```python
from build123d import *

# Parameters (mm, degrees)
SKETCH1_R                                      = 40
SKETCH1_R_2                                    = 20
BOSS_EXTRUDE1_DEPTH                            = 8.5
SKETCH2_R                                      = 1
CUT_EXTRUDE2_DEPTH                             = 58.203583804
SKETCH2_6_R                                    = 3
SKETCH2_6_R_2                                  = 1
BOSS_EXTRUDE3_DEPTH                            = 8.5
CIRPATTERN1_COUNT                              = 4
CUT_EXTRUDE4_DEPTH                             = 62.402361518
CIRPATTERN3_COUNT                              = 4
SKETCH7_R                                      = 21
CUT_EXTRUDE5_DEPTH                             = 7
SKETCH8_R                                      = 1
OUTER_RETAINER_M2_TAPPED_ENVELOPE_DEPTH        = 4.3
SKETCH9_R                                      = 1
REVB_OLDHAM_FOUR_M2_BLIND_THREAD_MAJOR_DEPTH   = 5.8
SKETCH10_R                                     = 1.51
REVB_OLDHAM_FOUR_D3P02_PILOT_POCKETS_DEPTH     = 1.1
SKETCH11_R                                     = 1.05
BENCH_OUTERRETAINER_M2_THREAD_MAJOR_ENVE_DEPTH = 4
SKETCH12_R                                     = 1.05
BENCH_OLDHAM_M2_CLEARANCE_4X_D2P1_DEPTH        = 9


with BuildPart() as part:
    # Sketch1 → Boss-Extrude1 (new body)
    with BuildSketch(Plane(origin=(0, 0, 0), x_dir=(1, 0, 0), z_dir=(0, 1, 0))):
        with Locations(Location((0, 0, 0), (0, 0, 270))):
            Circle(SKETCH1_R)
        with Locations(Location((0, 0, 0), (0, 0, 270))):
            Circle(SKETCH1_R_2, mode=Mode.SUBTRACT)
    extrude(amount=BOSS_EXTRUDE1_DEPTH)

    # Sketch2 → Cut-Extrude2 (cut, through all)
    with BuildSketch(Plane(origin=(0, 8.5, 0), x_dir=(1, 0, 0), z_dir=(0, 1, 0))):
        with Locations((40, 0)):
            Circle(SKETCH2_R)
    cut_extrude2 = extrude(amount=-CUT_EXTRUDE2_DEPTH, mode=Mode.SUBTRACT)

    # Sketch2_6 → Boss-Extrude3 (add)
    with BuildSketch(Plane(origin=(0, 8.5, 0), x_dir=(1, 0, 0), z_dir=(0, 1, 0))):
        with Locations((40, 0)):
            Circle(SKETCH2_6_R)
        with Locations(Location((40, 0, 0), (0, 0, 270))):
            Circle(SKETCH2_6_R_2, mode=Mode.SUBTRACT)
    boss_extrude3 = extrude(amount=-BOSS_EXTRUDE3_DEPTH)

    # CirPattern1: Cut-Extrude2, Boss-Extrude3 ×4 about axis
    cirpattern1_axis = Axis((0, 0, 0), (0, 1, 0))
    add([cut_extrude2.rotate(cirpattern1_axis, i * 360 / CIRPATTERN1_COUNT) for i in range(1, CIRPATTERN1_COUNT)], mode=Mode.SUBTRACT)
    add([boss_extrude3.rotate(cirpattern1_axis, i * 360 / CIRPATTERN1_COUNT) for i in range(1, CIRPATTERN1_COUNT)])

    # Sketch4 → Cut-Extrude4 (cut, through all)
    with BuildSketch(Plane(origin=(0, 8.5, 0), x_dir=(1, 0, 0), z_dir=(0, 1, 0))):
        with BuildLine():
            Line((-27.170578067, -25.049257724), (-17.377149148, -15.255828804))
            ThreePointArc((-17.377149148, -15.255828804), (-15.255828804, -15.255828804), (-15.255828804, -17.377149148))
            Line((-15.255828804, -17.377149148), (-25.049257724, -27.170578067))
            ThreePointArc((-25.049257724, -27.170578067), (-27.170578067, -27.170578067), (-27.170578067, -25.049257724))
        make_face()
    cut_extrude4 = extrude(amount=-CUT_EXTRUDE4_DEPTH, mode=Mode.SUBTRACT)

    # CirPattern3: Cut-Extrude4 ×4 about axis
    cirpattern3_axis = Axis((0, 0, 0), (0, 1, 0))
    for i in range(1, CIRPATTERN3_COUNT):
        add(cut_extrude4.rotate(cirpattern3_axis, i * 360 / CIRPATTERN3_COUNT), mode=Mode.SUBTRACT)

    # Sketch7 → Cut-Extrude5 (cut)
    with BuildSketch(Plane(origin=(0, 8.5, 0), x_dir=(1, 0, 0), z_dir=(0, 1, 0))):
        with Locations(Location((0, 0, 0), (0, 0, 270))):
            Circle(SKETCH7_R)
    extrude(amount=-CUT_EXTRUDE5_DEPTH, mode=Mode.SUBTRACT)

    # Sketch8 → Outer_Retainer_M2_Tapped_Envelope (cut)
    with BuildSketch(Plane(origin=(0, 8.5, 0), x_dir=(1, 0, 0), z_dir=(0, 1, 0))):
        with Locations(Location((0.720053396, -22.48847534, 0), (0, 0, 270))):
            Circle(SKETCH8_R)
        with Locations(Location((19.115564239, 11.867822203, 0), (0, 0, 270))):
            Circle(SKETCH8_R)
        with Locations(Location((-19.835617634, 10.620653137, 0), (0, 0, 270))):
            Circle(SKETCH8_R)
    extrude(amount=-OUTER_RETAINER_M2_TAPPED_ENVELOPE_DEPTH, mode=Mode.SUBTRACT)

    # Sketch9 → RevB_Oldham_Four_M2_Blind_Thread_Major (cut)
    with BuildSketch(Plane.XZ):
        with Locations(Location((27.716385975, 11.480502971, 0), (0, 0, 270))):
            Circle(SKETCH9_R)
        with Locations(Location((-11.480502971, 27.716385975, 0), (0, 0, 270))):
            Circle(SKETCH9_R)
        with Locations(Location((-27.716385975, -11.480502971, 0), (0, 0, 270))):
            Circle(SKETCH9_R)
        with Locations(Location((11.480502971, -27.716385975, 0), (0, 0, 270))):
            Circle(SKETCH9_R)
    extrude(amount=-REVB_OLDHAM_FOUR_M2_BLIND_THREAD_MAJOR_DEPTH, mode=Mode.SUBTRACT)

    # Sketch10 → RevB_Oldham_Four_D3p02_Pilot_Pockets (cut)
    with BuildSketch(Plane.XZ):
        with Locations(Location((27.716385975, 11.480502971, 0), (0, 0, 270))):
            Circle(SKETCH10_R)
        with Locations(Location((-11.480502971, 27.716385975, 0), (0, 0, 270))):
            Circle(SKETCH10_R)
        with Locations(Location((-27.716385975, -11.480502971, 0), (0, 0, 270))):
            Circle(SKETCH10_R)
        with Locations(Location((11.480502971, -27.716385975, 0), (0, 0, 270))):
            Circle(SKETCH10_R)
    extrude(amount=-REVB_OLDHAM_FOUR_D3P02_PILOT_POCKETS_DEPTH, mode=Mode.SUBTRACT)

    # Sketch11 → Bench_OuterRetainer_M2_Thread_Major_Enve (cut)
    with BuildSketch(Plane(origin=(0, 8.5, 0), x_dir=(1, 0, 0), z_dir=(0, 1, 0))):
        with Locations(Location((-22.37980351, -2.32258369, 0), (0, 0, 270))):
            Circle(SKETCH11_R)
        with Locations(Location((13.20131823, -18.22018653, 0), (0, 0, 270))):
            Circle(SKETCH11_R)
        with Locations(Location((9.17848528, 20.54277021, 0), (0, 0, 270))):
            Circle(SKETCH11_R)
    extrude(amount=-BENCH_OUTERRETAINER_M2_THREAD_MAJOR_ENVE_DEPTH, mode=Mode.SUBTRACT)

    # Sketch12 → Bench_Oldham_M2_Clearance_4x_D2p1 (cut)
    with BuildSketch(Plane(origin=(0, 8.5, 0), x_dir=(1, 0, 0), z_dir=(0, 1, 0))):
        with Locations(Location((27.71640367, -11.48048783, 0), (0, 0, 270))):
            Circle(SKETCH12_R)
        with Locations(Location((-11.48048527, -27.71637083, 0), (0, 0, 270))):
            Circle(SKETCH12_R)
        with Locations(Location((-27.71636828, 11.48051812, 0), (0, 0, 270))):
            Circle(SKETCH12_R)
        with Locations(Location((11.48052067, 27.71640112, 0), (0, 0, 270))):
            Circle(SKETCH12_R)
    extrude(amount=-BENCH_OLDHAM_M2_CLEARANCE_4X_D2P1_DEPTH, mode=Mode.SUBTRACT)


solid = part.part
```
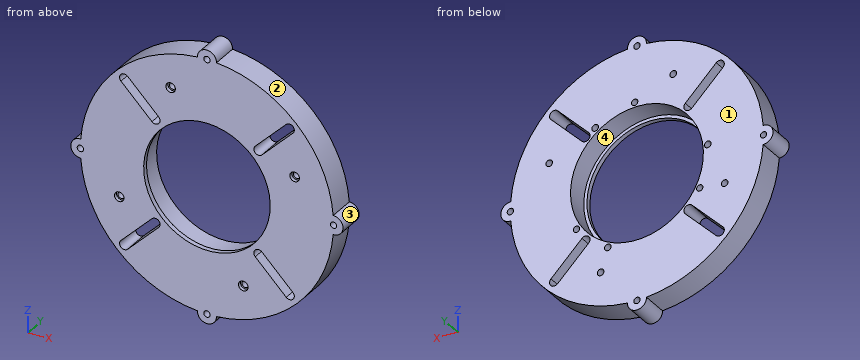
Design review of the part built by this model. Coordinates are the model's own, in mm. Face numbers are marked on the shaded views. Round coordinates to 2 decimals unless told otherwise and drop trailing zeros. Write each loop counter-clockwise with the first axis right and the second up, starting at its lowest first coordinate (ties: lowest second). Pieces come first, ordered by that corner, then holes.
Item 1: We need section B-B on y = 2.75. State how many separate pieces and enclosed holes the cut face has, and give its area (3 significant figures).
Item 2: The part is to be moulded in two halves that separate along Z. For the marked faces 1, 2, 3 and 4, say which applies: +Z half, -Z half, draft (parallel to the pull), parting line (faces both ways), or undercut.
Item 3: For probe 1 along X at (y, z) = (3, 0); probe 2 along Z at (x, y) = (-40, 2.75); probe 3 along X at (y, z) = (4.5, 16.5), list the stretches that pass through material, from the lowest coordinate up.
Item 4: Clearance check with flat-ended pins moving along their axes: pin 1 Ø5 at (y, z) = (3, -7.5) entering from -X; pin 2 Ø2.5 at (x, z) = (-27.72, -11.48) entering from -Y; pin 3 Ø0.6 at (x, z) = (9.5, -20.5) entering from +Y. State where each tip first meets the part, or that it passes through.
Item 5: We need section A-A on z = 0. Write out the cut boundary in (x, y), and give its area (3 significant figures).
Item 6: We need section C-C on x = -33. Write out the cut boundary in (y, z), and give its area (3 significant figures).
Returned:
1. separate pieces: 1
1. enclosed holes: 13
1. area: 3,480 mm2
2. face 1: draft
2. face 2: +Z half
2. face 3: parting line
2. face 4: undercut
3. probe 1: x = -43 to -41, -39 to -21, 21 to 39, 41 to 43
3. probe 2: z = -3 to -1, 1 to 3
3. probe 3: x = -36.44 to -18.62, -14.83 to -12.99, 12.99 to 14.83, 18.62 to 36.44
4. pin 1: stops at x = -39.69
4. pin 2: stops at y = 1.1
4. pin 3: stops at y = 4.5
5. outline: (-43, 0) - (-41, 0) - (-41, 8.5) - (-43, 8.5) - close; (-39, 0) - (-20, 0) - (-20, 1.5) - (-21, 1.5) - (-21, 8.5) - (-39, 8.5) - close; (20, 0) - (39, 0) - (39, 8.5) - (21, 8.5) - (21, 1.5) - (20, 1.5) - close; (41, 0) - (43, 0) - (43, 8.5) - (41, 8.5) - close
5. area: 343 mm2
6. outline: (0, -22.61) - (8.5, -22.61) - (8.5, 22.61) - (0, 22.61) - close
6. area: 384 mm2
